```python
from build123d import *

# Parameters (mm, degrees)
F0_R     = 19.05
F1_DEPTH = 15.875
F2_R     = 9.525
F3_DEPTH = 12.7
F5_R     = 1.5875
F6_DEPTH = 9.525
F7_R     = 1.5875
F8_DEPTH = 25.4


with BuildPart() as f1:
    # F0 (on Front) → F1 (new body)
    with BuildSketch(Plane.XZ):
        Circle(F0_R)
    extrude(amount=-F1_DEPTH)

    # F2 (on face) → F3 (cut)
    with BuildSketch(Plane.XZ):
        Circle(F2_R)
    extrude(amount=-F3_DEPTH, mode=Mode.SUBTRACT)

    # F5 (on face) → F6 (join)
    with BuildSketch(Plane.XZ.offset(-12.7)):
        Circle(F5_R)
    extrude(amount=-F6_DEPTH)

    # F7 (on face) → F8 (cut)
    with BuildSketch(Plane(origin=(0, 15.875, 0), x_dir=(-1, 0, 0), z_dir=(0, 1, 0))):
        with Locations((0, 6.35)):
            Circle(F7_R)
        with Locations((-4.490128, 4.490128)):
            Circle(F7_R)
        with Locations((-6.35, 0)):
            Circle(F7_R)
        with Locations((-4.490128, -4.490128)):
            Circle(F7_R)
        with Locations((0, -6.35)):
            Circle(F7_R)
        with Locations((4.490128, -4.490128)):
            Circle(F7_R)
        with Locations((6.35, 0)):
            Circle(F7_R)
        with Locations((4.490128, 4.490128)):
            Circle(F7_R)
    extrude(amount=-F8_DEPTH, mode=Mode.SUBTRACT)


solid = f1.part
```
Input: part model. Units: mm. Frame: model coordinates. A direction names the side the tool comes from. Give positions to 0.01 mm unless a question says otherwise; leave off trailing zeros. Order: outer loops, then holes, each group sorted by start corner. A loop starts at its lowest first (then second) coordinate and runs counter-clockwise, first axis right, second up. Notation, with made-up numbers: M 51,51.5 L 109,51.5 A29 ccw 109,89.5 Z; hole C 2.5,44 d1. An arc over 180 degrees is marked long. One line per question, with ' | ' between items.
1) Access query for faces 4 (the face through (0, 12.7, 0)), 5 (the face through (-0.73, 14.31, 4.94)). Directions: +Z, -Z, +X, -X, +Y, -Y. A direction counts if a zero-diameter tool reaches every point of the face in a straight line with its end or side. Return the directions, or none.
Filled in:
face 4: -Y | face 5: +Y, -Y
2) Ray query, L1, parallel to Z at x = 0, y = 13.5; L2, parallel to Y at x = 11.5, z = 11.5 (3 decimals); L3, parallel to Z at x = -1.5, y = 9.75. Return the intervals inside material, ascending.
Filled in:
L1: z = -19.05 to -7.94, -4.76 to 4.76, 7.94 to 19.05 | L2: y = 0 to 15.875 | L3: z = -18.99 to -9.41, 9.41 to 18.99
3) Section D-D on y = 5.75. Output: boundary loops of the cut face in (x, z) (3 decimals).
Filled in:
outline: C 0,0 d38.1; hole C 0,0 d19.05
4) Contact query for flat-ended pins moving along their axis: P1, Ø8, axis at x = -6.5, z = -7, coming from the +Y side (3 decimals); P2, Ø3.5, axis at x = -4.49, z = -4.49, coming from the -Y side; P3, Ø1, axis at x = -7, y = 15.5, coming from the +Z side. Output: stop coordinate, or through.
Filled in:
P1: stops at y = 15.875 | P2: stops at y = 12.7 | P3: stops at z = 17.91
5) Draft query along X for faces 1 (the face through (-0.34, 19.01, -1.55)), 2 (the face through (-4.764, 14.31, 0.07)), 3 (the face through (4, 0, 9)). Return one class per face: pulls with the +X half, pulls with the -X half, needs draft (parallel to the pull), parting line crosses it, or undercut.
Filled in:
face 1: parting line crosses it | face 2: undercut | face 3: needs draft
6) Section A-A on x = 0. State how many separate pieces and enclosed holes the cut face has, and give its area (3 significant figures).
Filled in:
separate pieces: 3 | enclosed holes: 0 | area: 363 mm2
